Read the model definition and answer for the solid it produces. Units are mm, in the model's axes. A direction names the side the tool comes from. Round coordinates to 2 decimals unless told otherwise and drop trailing zeros. Loops run counter-clockwise (first coordinate to the right, second up) from the corner with the lowest first, then second, coordinate; pieces in that order, holes last. Notation, with made-up numbers: (64.25, 10.5) - (85.25, 10.5) arc R26 ccw to (85.25, 24.5) - close; hole circle Ø11 at (3, 69). An arc over 180 degrees is marked (long way). Use one line per item in the form item = value. Start each with the question number.
```python
from build123d import *

# Parameters (mm, degrees)
EXTRUDE_1_DEPTH = 10
EXTRUDE_2_DEPTH = 16


with BuildPart() as part:
    # Эскиз1 → Повернуть1 (revolve)
    with BuildSketch(Plane.XY, mode=Mode.PRIVATE) as revolve_1_sk:
        Polygon((0, 0), (-48, 0), (-48, 2), (-50, 2), (-50, 8), (-20, 29), (-10, 29), (-10, 39), (-10, 136.5), (-7.5, 139), (0, 139), align=None)
    revolve(revolve_1_sk.sketch.rotate(Axis((0, 0, 0), (0, 1, 0)), 180), axis=Axis((0, 0, 0), (0, 1, 0)))  # turned: the seam where the file's is

    # Эскиз2 → Бобышка-Вытянуть1 (add)
    with BuildSketch(Plane(origin=(0, 29, 0), x_dir=(1, 0, 0), z_dir=(0, 1, 0))):
        Polygon((0, 17.320508076), (-15, 8.660254038), (-15, -8.660254038), (0, -17.320508076), (15, -8.660254038), (15, 8.660254038), align=None)
    extrude(amount=EXTRUDE_1_DEPTH)

    # Эскиз3 → Бобышка-Вытянуть2 (add)
    with BuildSketch(Plane(origin=(0, 87.75, 0), x_dir=(1, 0, 0), z_dir=(0, 1, 0))):
        Polygon((15, 8.660254038), (0, 17.320508076), (-15, 8.660254038), (-15, -8.660254038), (0, -17.320508076), (15, -8.660254038), align=None)
    extrude(amount=EXTRUDE_2_DEPTH)

    # Эскиз4 → Вырез-Повернуть2 (revolve, cut)
    with BuildSketch(Plane.XY, mode=Mode.PRIVATE) as cut_revolve_2_sk:
        Polygon((-28.856406461, 103.75), (-15, 103.75), (-28.856406461, 95.75), align=None)
        Polygon((-28.856406461, 87.75), (-28.856406461, 95.75), (-15, 87.75), align=None)
        Polygon((-23.660254038, 39), (-23.660254038, 34), (-15, 39), align=None)
        Polygon((-23.660254038, 34), (-23.660254038, 29), (-15, 29), align=None)
    revolve(cut_revolve_2_sk.sketch.rotate(Axis((0, 139, 0), (0, -1, 0)), 180), axis=Axis((0, 139, 0), (0, -1, 0)), mode=Mode.SUBTRACT)  # turned: the seam where the file's is


solid = part.part
```
1) For faces 1 (the conical face through (-13.45, 88.07, 7.81)), 2 (the flat face through (-15, 96, 0)), 3 (the conical face through (13.45, 88.07, -7.81)), determine the directions among +Z, -Z, +X, -X, +Y, -Y from which every point of the face is accessible in a straight line to the end or side of a thin tool.
2) A cutting plane is placed at A-A on y = 128. Write down the section's boundary in (x, z), plus the area to 3 significant figures.
3) Flat-ended cylindrical pins translate along their axes: pin 1 (3 mm diameter, centred on y = 35, z = 2.5, fed in from -X); pin 2 (1.5 mm diameter, centred on x = 3.5, y = 24.5, fed in from -Z); pin 3 (12 mm diameter, centred on x = 6, y = 28.5, fed in from +Z); pin 4 (4 mm diameter, centred on x = -36, z = 38, fed in from +Y). Find the tip coordinate at first contact, or state that the pin passes through.
4) A cutting plane is placed at B-B on y = 18. Write down the section's boundary in (x, z).
5) Straight lines are drawn through the part: line 1 (Y direction, x = 14.5, z = 6); line 2 (Z direction, x = -5, y = 54); line 3 (Y direction, x = -10.5, z = -12). For each, find the intervals that lie inside material, in ascending order. Write a range as from..to.
Checks:
q1.face_1 = +Z, -X
q1.face_2 = +Z, -Z, -X, +Y
q1.face_3 = -Z, +X
q2.outline = circle Ø20 at (0, 0)
q2.area = 314 mm²
q3.pin_1 = -15
q3.pin_2 = -27.28
q3.pin_3 = 28.74
q3.pin_4 = through
q4.outline = circle Ø71.43 at (0, 0)
q5.line_1 = 0..29, 29.4..38.6, 88.15..103.35
q5.line_2 = -8.66..8.66
q5.line_3 = 0..29
